Geometry check sheet. Reference: drawing and pictorial views, mm from the part's lowest x, y, z. A direction names the side the tool comes from. Round coordinates to 2 decimals unless told otherwise and drop trailing zeros. Order: outer loops, then holes, each group sorted by start corner. A loop starts at its lowest first (then second) coordinate and runs counter-clockwise, first axis right, second up.
Q1. Depth check by flat-ended pin: P1, Ø2, axis at y = 47, z = 27, coming from the -X side; P2, Ø12, axis at y = 27, z = 67, coming from the +X side; P3, Ø1, axis at y = 32, z = 68, coming from the -X side. Enter the tip coordinate at first touch or a pass-through.
Q2. Cross-section at B-B on z = 63. Record the cut outline in (x, y), then the cut area to 3 significant figures.
Q3. Cross-section at C-C on x = 59. Record the cut outline in (y, z).
Q4. Scan lines: probe 1 along Z at (x, y) = (56.5, 19); probe 2 along X at (y, z) = (33.5, 24) (1 decimal); probe 3 along Z at (x, y) = (39, 21). Record each from-to range of solid material in increasing order.
Q5. Mould release check, pull along X, two halves, no side actions. Record for the marked faces 1 and 2: +X half, -X half, draft (parallel to the pull), parting line (faces both ways), or undercut.
Q6. Cross-section at D-D on x = 82.5. Record the cut outline in (y, z).
Q7. Set-up check for the marked faces 3 and 4: record each of +Z, -Z, +X, -X, +Y, -Y from which the full face is reachable in a straight line by a thin tool's end or side.
Q8. Cross-section at A-A on y = 17.5. Record the cut outline in (x, z) (1 decimal).
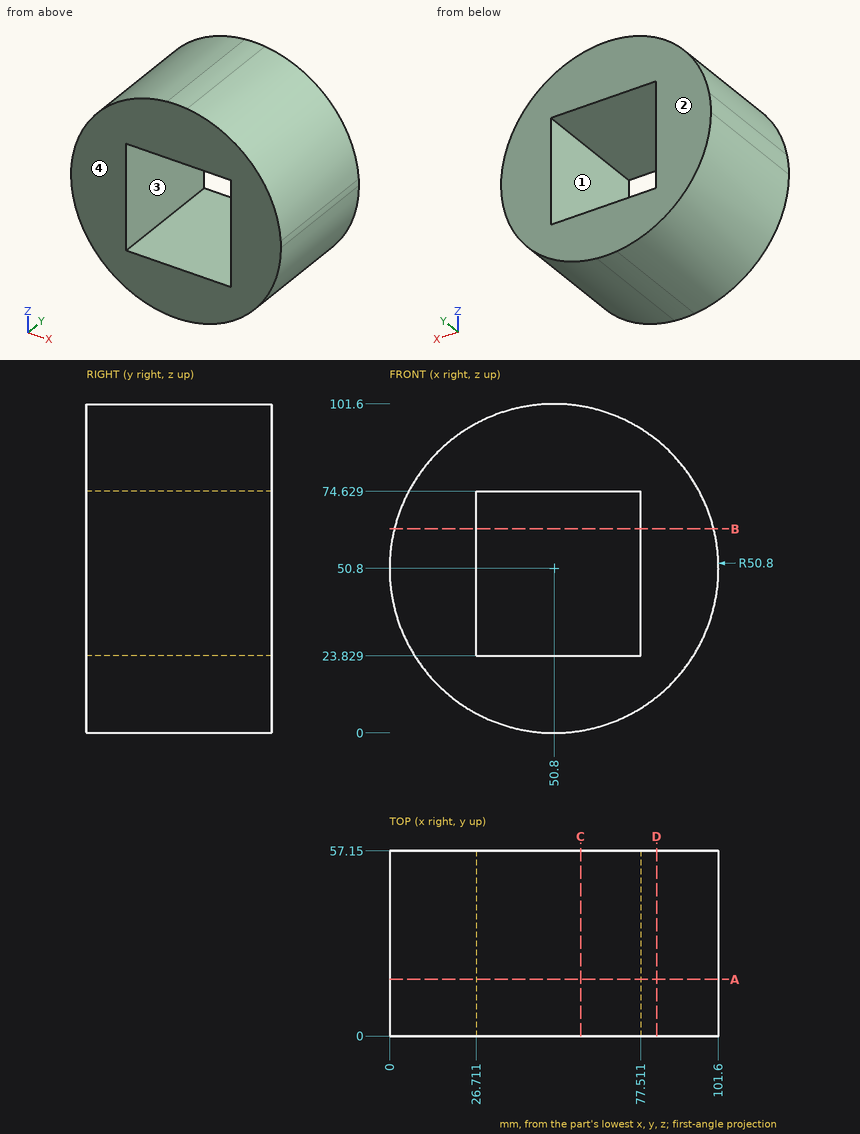
Results found:
1. P1: stops at x = 5.4
1. P2: stops at x = 100.57
1. P3: stops at x = 2.82
2. outline: (1.49, 0) - (26.71, 0) - (26.71, 57.15) - (1.49, 57.15) - close; (77.51, 0) - (100.11, 0) - (100.11, 57.15) - (77.51, 57.15) - close
2. area: 2,730 mm2
3. outline: (0, 0.67) - (57.15, 0.67) - (57.15, 23.83) - (0, 23.83) - close; (0, 74.63) - (57.15, 74.63) - (57.15, 100.93) - (0, 100.93) - close
4. probe 1: z = 0.32 to 23.83, 74.63 to 101.28
4. probe 2: x = 7.6 to 26.7, 77.5 to 94
4. probe 3: z = 1.39 to 23.83, 74.63 to 100.21
5. face 1: undercut
5. face 2: draft
6. outline: (0, 11.1) - (57.15, 11.1) - (57.15, 90.5) - (0, 90.5) - close
7. face 3: +Y, -Y
7. face 4: +Z, -Z, +X, -X, -Y
8. outline: circle Ø101.6 at (50.8, 50.8); hole (26.7, 23.8) - (77.5, 23.8) - (77.5, 74.6) - (26.7, 74.6) - close
